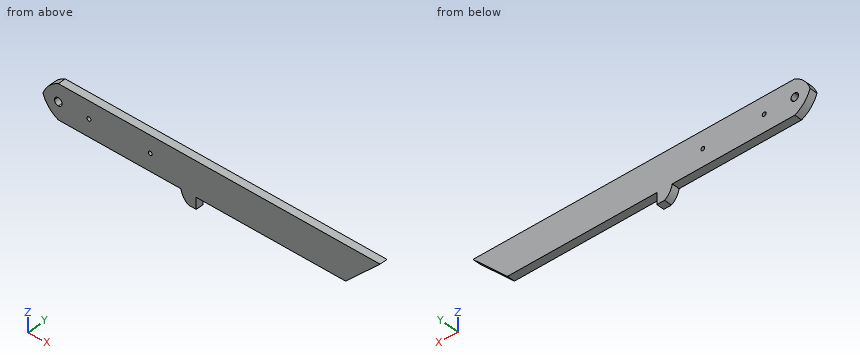
```python
from build123d import *

# Parameters (mm, degrees)
F1_DEPTH = 6.35


with BuildPart() as f1:
    # F0 (on Front) → F1 (new body)
    with BuildSketch(Plane.XZ):
        with BuildLine():
            Line((-127, 1.5875), (-127, -9.525))
            Line((-127, -9.525), (-25.4, -9.525))
            Line((-25.4, -9.525), (-25.4, 4.7625))
            Line((-25.4, 4.7625), (-49.2125, 4.7625))
            ThreePointArc((-49.2125, 4.7625), (-50.8, 3.175), (-52.3875, 4.7625))
            Line((-52.3875, 4.7625), (-100.0125, 4.7625))
            ThreePointArc((-100.0125, 4.7625), (-101.6, 3.175), (-103.1875, 4.7625))
            Line((-103.1875, 4.7625), (-123.825, 4.7625))
            ThreePointArc((-123.825, 4.7625), (-124.7549359697, 2.5174359697), (-127, 1.5875))
        make_face()
        with BuildLine():
            Line((-25.4, 19.05), (-127, 19.05))
            Line((-127, 19.05), (-127, 7.9375))
            ThreePointArc((-127, 7.9375), (-124.7549359697, 7.0075640303), (-123.825, 4.7625))
            Line((-123.825, 4.7625), (-103.1875, 4.7625))
            ThreePointArc((-103.1875, 4.7625), (-101.6, 6.35), (-100.0125, 4.7625))
            Line((-100.0125, 4.7625), (-52.3875, 4.7625))
            ThreePointArc((-52.3875, 4.7625), (-50.8, 6.35), (-49.2125, 4.7625))
            Line((-49.2125, 4.7625), (-25.4, 4.7625))
            Line((-25.4, 4.7625), (-25.4, 19.05))
        make_face()
        with BuildLine():
            Line((-127, 7.9375), (-127, 19.05))
            ThreePointArc((-127, 19.05), (-134.856835688, 13.2456595004), (-139.7, 4.7625))
            Line((-139.7, 4.7625), (-130.175, 4.7625))
            ThreePointArc((-130.175, 4.7625), (-129.2450640303, 7.0075640303), (-127, 7.9375))
        make_face()
        with BuildLine():
            Line((-130.175, 4.7625), (-139.7, 4.7625))
            ThreePointArc((-139.7, 4.7625), (-134.856835688, -3.7206595004), (-127, -9.525))
            Line((-127, -9.525), (-127, 1.5875))
            ThreePointArc((-127, 1.5875), (-129.2450640303, 2.5174359697), (-130.175, 4.7625))
        make_face()
        Polygon((-12.7, 19.05), (-19.05, 19.05), (-19.05, -19.05), (-12.7, -19.05), (-12.7, -9.525), (-12.7, 4.7625), align=None)
        with BuildLine():
            Line((-19.05, 19.05), (-25.4, 19.05))
            Line((-25.4, 19.05), (-25.4, 4.7625))
            Line((-25.4, 4.7625), (-25.4, -9.525))
            ThreePointArc((-25.4, -9.525), (-23.3236183324, -15.0199122216), (-19.05, -19.05))
            Line((-19.05, -19.05), (-19.05, 19.05))
        make_face()
        Polygon((139.7, 19.05), (119.4944237276, 19.05), (105.2069237276, 4.7625), (-12.7, 4.7625), (-12.7, -9.525), (111.125, -9.525), align=None)
        Polygon((119.4944237276, 19.05), (-12.7, 19.05), (-12.7, 4.7625), (105.2069237276, 4.7625), align=None)
    extrude(amount=F1_DEPTH)


solid = f1.part
```
Verification items for the finished model (mm, model axes). Give positions to 0.01 mm unless a question says otherwise; leave off trailing zeros. Loops run counter-clockwise (first coordinate to the right, second up) from the corner with the lowest first, then second, coordinate; pieces in that order, holes last.
1. Section check C-C, the plane z = -4.5. Enter the section's corners in (x, y), then the cut area to 3 significant figures.
2. Thickness scan on line 1 (Z direction, x = -101.6, y = -3.5) (3 decimals); line 2 (Z direction, x = -32.5, y = -2.5) (3 decimals). Record the ranges inside material, lowest first.
3. Section check B-B, the plane x = -119.5. Enter the section's corners in (y, z) (3 decimals), then the cut area to 3 significant figures.
4. Go/stop test with flat-tipped pins: pin 1 Ø1.9 at (x, y) = (-65, -4) entering from -Z (3 decimals); pin 2 Ø4 at (x, z) = (-101.6, 4.76) entering from -Y; pin 3 Ø1.5 at (y, z) = (-2, -1) entering from -X. Record where each tip stops, or that it passes through.
5. Section check A-A, the plane y = -3.5. Count the separate pieces of the cut face and the enclosed holes in it, then the cut area to 3 significant figures.
Geometry says:
1. outline: (-134.13, -6.35) - (116.15, -6.35) - (116.15, 0) - (-134.13, 0) - close
1. area: 1,590 mm2
2. line 1: z = -9.525 to 3.175, 6.35 to 19.05
2. line 2: z = -9.525 to 19.05
3. outline: (-6.35, -9.525) - (0, -9.525) - (0, 19.05) - (-6.35, 19.05) - close
3. area: 181 mm2
4. pin 1: stops at z = -9.525
4. pin 2: stops at y = -6.35
4. pin 3: stops at x = -137.42
5. separate pieces: 1
5. enclosed holes: 3
5. area: 7,500 mm2
